CAD build for the part. Positions are in the model's coordinates, mm. A direction names the side the tool comes from. Coordinates: 2 decimals unless noted, no trailing zeros.
Autodesk Inventor part; units mm, degrees
ref_plane "YZ Plane" through (0, 0, 0) normal (1, 0, 0) x (0, 1, 0)
ref_plane "XZ Plane" through (0, 0, 0) normal (0, 1, 0) x (-1, 0, 0)
ref_plane "XY Plane" through (0, 0, 0) normal (0, 0, 1) x (1, 0, 0)
sketch "Sketch3" plane through (0, 0, 0) normal (0, 0, 1) x (1, 0, 0)
  line L0 (-80.5781, 0.8246) -> (-80.5781, 20.7988) construction
  circle A0 centre (-80.5781, 0.8246) radius 13.481
  line L1 (-53.7179, 12.5571) -> (-53.7179, -10.9927)
  arc A1 (-53.7179, -10.9927) -> (-51.5054, -12.9814) centre (-51.7179, -10.9927) ccw
  arc A2 (-51.5054, 14.5458) -> (-53.7179, 12.5571) centre (-51.7179, 12.5571) ccw
  line L2 (36.2229, -3.6088) -> (-51.5054, -12.9814)
  line L3 (38.0104, 3.1845) -> (38.0104, -1.6201)
  line L4 (-80.5781, 0.8246) -> (49.5525, 0.8246) construction
  circle A3 centre (49.6953, -3.8247) radius 5.6609
  line L5 (59.6953, 14.884) -> (59.6953, -12.7998) construction
  spline S0 degree 4 poles (77.9414, 11.0338) (75.5683, 12.9654) (71.7145, 13.0272) (66.8099, 13.9036) (60.7685, 14.7338) (56.2959, 15.3578) (51.7728, 15.9509) (47.2242, 16.5426) (42.6244, 17.1111) (37.9974, 17.6651) (33.3378, 18.1987) (28.6546, 18.7114) (23.9504, 19.2026) (19.2309, 19.6699) (14.5002, 20.1135) (9.7632, 20.5291) (5.025, 20.9191) (0.2903, 21.2792) (-4.4372, 21.6095) (-9.151, 21.9092) (-13.8524, 22.1766) (-18.5268, 22.4102) (-23.2002, 22.6105) (-27.8558, 22.7627) (-32.4748, 22.8704) (-37.0553, 22.9312) (-41.5904, 22.9454) (-46.0738, 22.9127) (-50.5027, 22.8323) (-54.8678, 22.7052) (-59.1755, 22.5324) (-63.394, 22.3084) (-67.5752, 22.0492) (-71.5451, 21.7209) (-75.7777, 21.4072) (-79.04, 20.9063) (-83.4863, 20.5541) (-87.0067, 20.037) (-90.7113, 19.5168) (-94.2172, 18.9459) (-97.6363, 18.3426) (-100.9342, 17.7015) (-104.1216, 17.0263) (-107.1909, 16.3187) (-110.1396, 15.5797) (-112.9656, 14.8117) (-115.6652, 14.0172) (-118.2357, 13.1965) (-120.6759, 12.3541) (-122.9817, 11.4895) (-125.1529, 10.6071) (-127.1857, 9.7065) (-129.0794, 8.7914) (-130.8324, 7.8633) (-132.4429, 6.923) (-133.9096, 5.9737) (-135.2322, 5.016) (-136.4083, 4.0508) (-137.4392, 3.0816) (-138.3215, 2.1025) (-139.0592, 1.1321) (-139.6407, 0.1249) (-140.106, -0.8362) (-140.3589, -2.0477) (-140.602, -2.598) (-140.1166, -5.4607) (-140.0539, -5.4622) (-139.4639, -6.7645) (-138.8842, -7.4979) (-138.1173, -8.3934) (-137.2199, -9.1877) (-136.1721, -9.9852) (-134.9893, -10.738) (-133.6669, -11.4655) (-132.2091, -12.1599) (-130.6156, -12.8245) (-128.8897, -13.4579) (-127.0312, -14.0591) (-125.0439, -14.6296) (-122.9287, -15.1678) (-120.6879, -15.6738) (-118.3241, -16.1476) (-115.8396, -16.5892) (-113.2366, -16.9984) (-110.5176, -17.3742) (-107.6861, -17.7183) (-104.7439, -18.0297) (-101.6943, -18.3095) (-98.5398, -18.5568) (-95.2843, -18.7732) (-91.9297, -18.9579) (-88.48, -19.1131) (-84.9381, -19.2376) (-81.3071, -19.3341) (-77.5906, -19.4015) (-73.7915, -19.4421) (-69.9139, -19.4561) (-65.961, -19.445) (-61.9362, -19.4102) (-57.8434, -19.3518) (-53.6861, -19.2727) (-49.4679, -19.1731) (-45.1932, -19.0538) (-40.8649, -18.9183) (-36.4879, -18.766) (-32.0649, -18.5992) (-27.598, -18.4192) (-23.0941, -18.227) (-18.5434, -18.0273) (-13.9382, -17.8076) (-9.3141, -17.5719) (-4.666, -17.3195) (-0.0002, -17.052) (4.6675, -16.7728) (9.3655, -16.4759) (14.0236, -16.1832) (19.545, -15.7815) (23.3079, -15.6072) (27.1098, -15.1781) (28.8959, -15.0599) knots 0 0 0 0 0 0.024672 0.034555 0.0445 0.054495 0.064543 0.074632 0.084755 0.094911 0.105094 0.115299 0.125521 0.135755 0.145995 0.156237 0.166475 0.176705 0.186921 0.197118 0.207299 0.217463 0.227605 0.23772 0.247796 0.257824 0.267798 0.277713 0.287563 0.297345 0.307053 0.31668 0.326224 0.335555 0.344908 0.354162 0.363308 0.372467 0.381393 0.390196 0.398872 0.407415 0.41582 0.424082 0.432193 0.44015 0.447945 0.455574 0.46303 0.470307 0.477401 0.484305 0.491015 0.497525 0.503831 0.509931 0.515822 0.521506 0.526986 0.53227 0.537373 0.542316 0.547131 0.552525 0.557529 0.562533 0.567581 0.57205 0.576988 0.582082 0.587354 0.592817 0.598478 0.604341 0.610406 0.616671 0.623133 0.629789 0.636632 0.643658 0.650861 0.658236 0.665777 0.673478 0.681333 0.689338 0.697486 0.705771 0.71419 0.722736 0.731403 0.740188 0.749084 0.758087 0.767192 0.776393 0.785687 0.795067 0.804529 0.814069 0.823682 0.833362 0.843106 0.852907 0.862763 0.872667 0.88262 0.892624 0.902675 0.912766 0.92289 0.933033 0.943191 0.953358 0.963531 0.973703 0.984092 1 1 1 1 1
  line L6 (7.5013, -16.4763) -> (50.2906, -13.6435) construction
  arc A4 (44.8353, -17.2546) -> (13.385, -19.3367) centre (31.5327, -54.8885) ccw construction
  line L7 (159.6953, -3.8066) -> (59.6953, -3.8066) construction
  line L8 (-51.5054, 14.5458) -> (36.2229, 5.1732)
  arc A5 (36.2229, -3.6088) -> (38.0104, -1.6201) centre (36.0104, -1.6201) ccw
  arc A6 (38.0104, 3.1845) -> (36.2229, 5.1732) centre (36.0104, 3.1845) ccw
  spline S1 degree 4 poles (78.1029, 11.0141) (76.6463, 11.2227) (73.9909, 10.5042) (70.2765, 8.6041) (66.0429, 5.3938) (62.3889, 1.8499) (60.314, -1.2467) (59.5572, -3.5763) (59.5773, -5.0793) knots 0 0 0 0 0 0.302475 0.43895 0.576633 0.708802 1 1 1 1 1
  spline S2 degree 4 poles (28.8959, -15.0599) (34.0984, -14.7105) (49.269, -14.182) (58.5645, -15.239) (59.5773, -5.0793) knots 0 0 0 0 0 1 1 1 1 1
  line L9 (28.8959, -15.0599) -> (34.0984, -14.7105) construction
  line L10 (34.0984, -14.7105) -> (49.269, -14.182) construction
  line L11 (49.269, -14.182) -> (58.5645, -15.239) construction
  line L12 (58.5645, -15.239) -> (59.5773, -5.0793) construction
  line L13 (-140.4646, -2.8394) -> (159.4818, -3.8173) construction
  line L14 (-132.0856, 0.6333) -> (-132.0856, -6.3667)
  line L15 (-132.0856, -6.3667) -> (-110.3816, -12.3574)
  line L16 (-110.3816, -12.3574) -> (-104.797, -12.3574)
  line L17 (-104.797, -12.3574) -> (-104.797, -18.0156)
  line L18 (-132.0856, 0.6333) -> (-110.3816, 10.553)
  line L19 (-110.3816, 10.553) -> (-104.1736, 10.553)
  line L20 (-104.1736, 10.553) -> (-104.1736, 17.0026)
  line L21 (38.0104, 0.8246) -> (38.0104, -14.6534)
  line L22 (38.0104, 0.8246) -> (38.0104, 17.6585)
  point P0 (0, 0)
  point P1 (17.6589, 23.5628)
  point P2 (75.883, 10.8572)
  point P3 (72.8647, 9.7686)
  point P4 (69.4179, 7.8149)
  point P5 (66.0452, 5.2617)
  point P6 (63.1887, 2.4463)
  point P7 (61.1228, -0.3317)
  point P8 (59.9357, -2.8689)
  point P9 (-160.0931, -3.8671)
  point P10 (28.8959, -15.0599)
  point P11 (69.5533, 13.4647)
  point P12 (65.1899, 14.1023)
  point P13 (60.7936, 14.7318)
  point P14 (56.3207, 15.3468)
  point P15 (51.7945, 15.947)
  point P16 (47.2398, 16.5346)
  point P17 (42.6414, 17.1053)
  point P18 (33.3491, 18.1925)
  point P19 (28.6632, 18.7055)
  point P20 (23.9568, 19.1966)
  point P21 (19.2348, 19.6643)
  point P22 (14.5017, 20.1074)
  point P23 (9.7623, 20.5238)
  point P24 (5.0217, 20.9132)
  point P25 (0.2844, 21.2735)
  point P26 (-4.4451, 21.6038)
  point P27 (-9.1614, 21.9032)
  point P28 (-13.86, 22.1702)
  point P29 (-18.5361, 22.4036)
  point P30 (-23.211, 22.601)
  point P31 (-27.8721, 22.754)
  point P32 (-32.4966, 22.8611)
  point P33 (-37.0797, 22.9217)
  point P34 (-41.6169, 22.9356)
  point P35 (-46.1028, 22.9023)
  point P36 (-50.5329, 22.8216)
  point P37 (-54.9021, 22.6941)
  point P38 (-59.2065, 22.5195)
  point P39 (-63.4406, 22.2977)
  point P40 (-67.6008, 22.0302)
  point P41 (-71.6806, 21.7165)
  point P42 (-75.6814, 21.3591)
  point P43 (-79.1834, 20.9458)
  point P44 (-83.4048, 20.5095)
  point P45 (-87.1309, 20.023)
  point P46 (-90.7527, 19.494)
  point P47 (-94.2725, 18.9266)
  point P48 (-97.6845, 18.3211)
  point P49 (-100.9861, 17.6791)
  point P50 (-107.2438, 16.2934)
  point P51 (-110.1931, 15.553)
  point P52 (-113.0194, 14.7835)
  point P53 (-115.7191, 13.987)
  point P54 (-118.2898, 13.165)
  point P55 (-120.7294, 12.3201)
  point P56 (-123.0349, 11.454)
  point P57 (-125.2048, 10.569)
  point P58 (-127.2364, 9.6666)
  point P59 (-129.1282, 8.7491)
  point P60 (-130.8786, 7.8185)
  point P61 (-132.486, 6.8762)
  point P62 (-133.9488, 5.9245)
  point P63 (-135.2661, 4.9648)
  point P64 (-136.4363, 3.9987)
  point P65 (-137.4592, 3.0275)
  point P66 (-138.3336, 2.0531)
  point P67 (-139.0591, 1.0763)
  point P68 (-139.6352, 0.0983)
  point P69 (-140.0613, -0.8802)
  point P70 (-140.338, -1.8576)
  point P71 (-140.1239, -5.2398)
  point P72 (-139.9547, -5.7022)
  point P73 (-139.492, -6.6066)
  point P74 (-138.8844, -7.4823)
  point P75 (-138.1328, -8.3292)
  point P76 (-137.2384, -9.147)
  point P77 (-136.202, -9.9355)
  point P78 (-135.0249, -10.6943)
  point P79 (-133.7085, -11.4228)
  point P80 (-132.2548, -12.1206)
  point P81 (-130.6648, -12.7879)
  point P82 (-128.941, -13.4239)
  point P83 (-127.0846, -14.0282)
  point P84 (-125.0983, -14.6009)
  point P85 (-122.9839, -15.1415)
  point P86 (-120.7435, -15.6497)
  point P87 (-118.3798, -16.1256)
  point P88 (-115.8952, -16.569)
  point P89 (-113.2918, -16.9797)
  point P90 (-110.5723, -17.3574)
  point P91 (-107.74, -17.7027)
  point P92 (-101.7463, -18.2964)
  point P93 (-98.5909, -18.5451)
  point P94 (-95.3341, -18.7623)
  point P95 (-91.9783, -18.9484)
  point P96 (-88.5271, -19.1041)
  point P97 (-84.9838, -19.2298)
  point P98 (-81.3514, -19.3267)
  point P99 (-77.6332, -19.3951)
  point P100 (-73.8324, -19.4362)
  point P101 (-69.9531, -19.4509)
  point P102 (-65.9985, -19.4404)
  point P103 (-61.9719, -19.4059)
  point P104 (-57.8772, -19.3483)
  point P105 (-53.718, -19.2694)
  point P106 (-49.4979, -19.1701)
  point P107 (-45.2211, -19.0516)
  point P108 (-40.8909, -18.916)
  point P109 (-36.5118, -18.7642)
  point P110 (-32.0871, -18.5977)
  point P111 (-27.6213, -18.418)
  point P112 (-23.1183, -18.2269)
  point P113 (-18.5646, -18.0247)
  point P114 (-13.9566, -17.8054)
  point P115 (-9.3252, -17.5693)
  point P116 (-4.674, -17.317)
  point P117 (-0.0078, -17.05)
  point P118 (4.6686, -16.7695)
  point P119 (9.3513, -16.477)
  point P120 (14.0352, -16.1731)
  point P121 (18.7161, -15.8596)
  point P122 (23.3889, -15.5371)
  point P123 (78.0825, 12.164)
  point P124 (159.2574, -3.8401)
  point P125 (158.8836, -3.8779)
  point P126 (158.3607, -3.9307)
  point P127 (157.6896, -3.9985)
  point P128 (156.8706, -4.081)
  point P129 (155.9046, -4.1779)
  point P130 (154.7931, -4.2892)
  point P131 (153.5367, -4.4143)
  point P132 (152.1372, -4.5532)
  point P133 (150.5955, -4.7056)
  point P134 (148.914, -4.8712)
  point P135 (147.0936, -5.0494)
  point P136 (145.137, -5.2399)
  point P137 (143.0457, -5.4421)
  point P138 (140.8221, -5.6563)
  point P139 (138.4686, -5.8813)
  point P140 (135.9876, -6.1174)
  point P141 (133.3815, -6.3634)
  point P142 (130.6533, -6.6196)
  point P143 (127.8054, -6.8851)
  point P144 (124.8414, -7.1596)
  point P145 (121.7634, -7.4428)
  point P146 (118.5756, -7.7341)
  point P147 (115.2804, -8.0332)
  point P148 (111.8817, -8.3395)
  point P149 (108.3828, -8.6527)
  point P150 (104.787, -8.9722)
  point P151 (101.0985, -9.2974)
  point P152 (97.3206, -9.6283)
  point P153 (93.4572, -9.9643)
  point P154 (89.5122, -10.3048)
  point P155 (85.4898, -10.6492)
  point P156 (81.3936, -10.9969)
  point P157 (77.2284, -11.3479)
  point P158 (72.9975, -11.701)
  point P159 (68.7057, -12.0556)
  point P160 (64.3572, -12.4117)
  point P161 (59.9559, -12.7678)
  point P162 (55.5069, -13.1239)
  point P163 (51.0138, -13.4788)
  point P164 (46.4817, -13.8316)
  point P165 (41.9148, -14.182)
  point P166 (35.7035, -14.3277)
  point P167 (32.6946, -14.8708)
  point P168 (82.2459, 11.5043)
  point P169 (86.3364, 10.8401)
  point P170 (90.3495, 10.1732)
  point P171 (94.2816, 9.5051)
  point P172 (98.1288, 8.837)
  point P173 (101.8872, 8.171)
  point P174 (105.5538, 7.5086)
  point P175 (109.1244, 6.8507)
  point P176 (112.596, 6.1997)
  point P177 (115.9653, 5.5565)
  point P178 (119.2287, 4.9229)
  point P179 (122.3835, 4.3007)
  point P180 (125.4264, 3.6911)
  point P181 (128.3547, 3.0956)
  point P182 (131.1654, 2.5157)
  point P183 (133.8561, 1.9532)
  point P184 (136.4244, 1.4093)
  point P185 (138.8676, 0.8855)
  point P186 (141.1833, 0.383)
  point P187 (143.3697, -0.0964)
  point P188 (145.4247, -0.5518)
  point P189 (147.3462, -0.9817)
  point P190 (149.1327, -1.3852)
  point P191 (150.7821, -1.7608)
  point P192 (152.2935, -2.1073)
  point P193 (153.6651, -2.4241)
  point P194 (154.8954, -2.7103)
  point P195 (155.9838, -2.9647)
  point P196 (156.9291, -3.187)
  point P197 (157.7307, -3.376)
  point P198 (158.3871, -3.5317)
  point P199 (158.8986, -3.6529)
  dimension "d3" = 26.962
  dimension "d6" = 11.3219
  dimension "d7" = 110
  dimension "d8" = 100
  dimension "d9" = 2
  dimension "d11" = 4.6493
  dimension "d25" = 7
  dimension "d26" = 3.5
  dimension "d27" = 8.379
  dimension "d28" = 30.083
  dimension "d29" = 5
  dimension "d30" = 5
  dimension "d31" = 59.8865
extrude "Extrusion3" add sketch "Sketch3" along normal blind 74.75 contours L22 S0 S1 S2 L21 L3
sketch "Sketch4" plane through (0, 0, 74.75) normal (0, 0, 1) x (1, 0, 0)
  circle A0 centre (49.6953, -3.8247) radius 5.6609
  line L0 (44.0343, -3.8247) -> (38.0104, -3.8247) construction
  line L1 (38.0104, 17.6585) -> (38.0104, -14.6534)
  line L2 (45.5024, -4.8247) -> (36.5424, -4.8247)
  line L3 (36.5424, -4.8247) -> (36.5424, -2.8247)
  line L4 (36.5424, -2.8247) -> (45.5024, -2.8247)
  line L5 (45.5024, -2.8247) -> (45.5024, -4.8247)
  line L6 (45.5024, -4.8247) -> (36.5424, -2.8247) construction
  line L7 (36.5424, -4.8247) -> (45.5024, -2.8247) construction
  point P0 (0, 0)
  point P1 (41.0224, -3.8247)
  dimension "d34" = 8.96
  dimension "d35" = 2
extrude "Extrusion4" cut sketch "Sketch4" against normal blind 103.75 contours L4 L5 L2 A0 | A0 L2 L1 L4 | L1 L2 L3 L4 picked at (45.0164, -3.9363)
properties part number "4P.01.01.11-TW-v1-WingRibWFlapSingle" material "Polyurethane Foam"
1) Which spindle directions (+Z, -Z, +X, -X, +Y, -Y) get a long thin tool onto all of the face, cutting with end or side? Do faces 1 (the flat face through (41, -4.825, 38)), 2 (the flat face through (53, 5, 74.75)). Say none if no direction does.
2) Pin check, flat tips, straight feed: P1, Ø12, axis at x = 62, z = 10.5, coming from the +Y side; P2, Ø4, axis at x = 61, z = 67.5, coming from the +Y side; P3, Ø12, axis at x = 69.5, z = 37, coming from the -Y side. Stop position of each tip, or through.
3) Drill centre lines: probe 1 along X at (y, z) = (-8, 33); probe 2 along Y at (x, z) = (44, 27); probe 3 along Y at (x, z) = (49, 20.5). Where is each one in solid material? Low to high.
4) Two-plate mould, pull along Y, no slides. Class faces 3 (the flat face through (38.01, -10, 37)), 4 (the flat face through (41, -2.825, 38)): released by +Y, released by -Y, zero draft, split by the parting line, or undercut.
Worked out:
1. face 1: +Z, -Z, -X
1. face 2: +Z, +X, -X, +Y, -Y
2. P1: stops at y = 15.39
2. P2: stops at y = 14.98
2. P3: stops at y = 2.79
3. probe 1: x = 38.01 to 45.87, 53.52 to 58.91
3. probe 2: y = -14.35 to -4.82, -2.82 to 16.94
3. probe 3: y = -13.83 to -9.44, 1.79 to 16.31
4. face 3: zero draft
4. face 4: undercut
